Can you work these out from the drawing? Everything is in mm from the part's minimum corner. Coordinates: 2 decimals unless noted, no trailing zeros. Loops run counter-clockwise (first coordinate to the right, second up) from the corner with the lowest first, then second, coordinate; pieces in that order, holes last. Notation, with made-up numbers: (47.25, -13.5) -> (73.25, -13.5) arc R19 ccw to (73.25, -5.5) -> close; hole circle Ø6 at (31, 37). An arc over 180 degrees is marked (long way). Put each result on its own line as item: value. Start each with the question number.
Item 1: If we section it at A-A on y = 11: Please give me the cut outline in (x, z).
Item 2: If we section it at C-C on y = 17: Please give me the cut outline in (x, z) (1 decimal), plus the area to 3 significant figures.
Item 3: We'd pull the mould along X, two halves only. Please class the marked faces 1, 2 and 3: pulls with the +X half, pulls with the -X half, needs draft (parallel to the pull), parting line crosses it, or undercut.
Item 4: Will these pins go through, and if not, where does the flat tip stop? P1, Ø1.5, axis at x = 5.34, y = 5.34, coming from the +Z side; P2, Ø2, axis at x = 5, z = 1, coming from the -Y side; P3, Ø3, axis at x = 15.5, z = 1, coming from the -Y side; P4, Ø3, axis at x = 19, z = 3, coming from the -Y side.
Item 5: If we section it at D-D on x = 2.25: Please give me the cut outline in (y, z).
Item 6: Please list where these lines run through material, in increasing order: L1, parallel to Y at x = 11, z = 3.25; L2, parallel to X at y = 5.25, z = 7; L3, parallel to Y at x = 6, z = 6.25. Write a range as from..to.
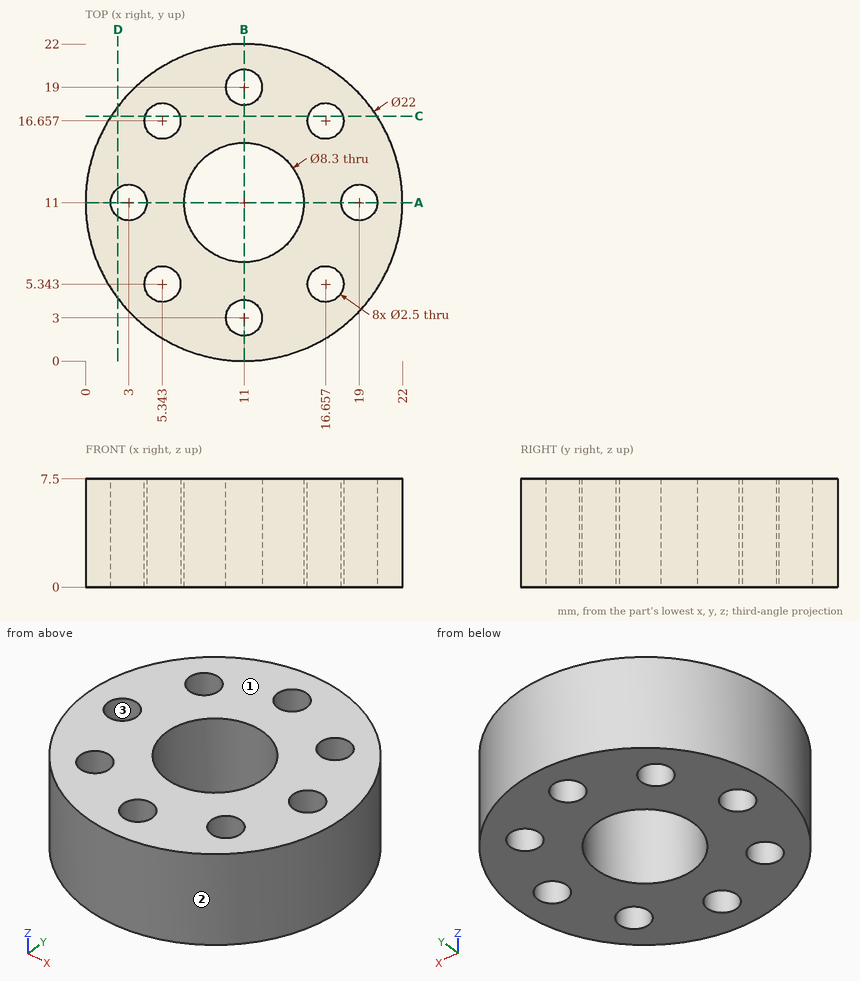
Solutions:
1. outline: (0, 0) -> (1.75, 0) -> (1.75, 7.5) -> (0, 7.5) -> close; (4.25, 0) -> (6.85, 0) -> (6.85, 7.5) -> (4.25, 7.5) -> close; (15.15, 0) -> (17.75, 0) -> (17.75, 7.5) -> (15.15, 7.5) -> close; (20.25, 0) -> (22, 0) -> (22, 7.5) -> (20.25, 7.5) -> close
2. outline: (1.8, 0) -> (4.1, 0) -> (4.1, 7.5) -> (1.8, 7.5) -> close; (6.5, 0) -> (15.5, 0) -> (15.5, 7.5) -> (6.5, 7.5) -> close; (17.9, 0) -> (20.2, 0) -> (20.2, 7.5) -> (17.9, 7.5) -> close
2. area: 102 mm^2
3. face 1: needs draft
3. face 2: parting line crosses it
3. face 3: undercut
4. P1: through
4. P2: y = 1.2
4. P3: y = 0.42
4. P4: y = 2.13
5. outline: (4.33, 0) -> (10, 0) -> (10, 7.5) -> (4.33, 7.5) -> close; (12, 0) -> (17.67, 0) -> (17.67, 7.5) -> (12, 7.5) -> close
6. L1: 0..1.75, 4.25..6.85, 15.15..17.75, 20.25..22
6. L2: 1.62..4.1, 6.59..15.41, 17.9..20.38
6. L3: 1.2..4.28, 6.41..15.59, 17.72..20.8
